Part model, mm, in its own coordinate system. Round coordinates to 2 decimals unless told otherwise and drop trailing zeros. Loops run counter-clockwise (first coordinate to the right, second up) from the corner with the lowest first, then second, coordinate; pieces in that order, holes last. Notation, with made-up numbers: (83, 28) - (98, 28) arc R19 cw to (98, 57) - close; hole circle Ø8 at (-5.75, 17.5). An arc over 180 degrees is marked (long way). Put each result on its own line as item: value.
from build123d import *

# Parameters (mm, degrees)
SKETCH_1_W          = 65
SKETCH_1_H          = 105
EXTRUDE_1_DEPTH     = 3
SKETCH_2_R          = 1.4
CUT_EXTRUDE_1_DEPTH = 62.818282085
SKETCH_3_R          = 1.4
CUT_EXTRUDE_2_DEPTH = 62.818282085
SKETCH_6_R          = 1.5
CUT_EXTRUDE_5_DEPTH = 62.818282085


with BuildPart() as part:
    # 草图1 → 凸台-拉伸1 (new body)
    with BuildSketch(Plane(origin=(0, 0, 0), x_dir=(1, 0, 0), z_dir=(0, 1, 0))):
        Rectangle(SKETCH_1_W, SKETCH_1_H)
    extrude(amount=EXTRUDE_1_DEPTH)

    # 草图2 → 切除-拉伸1 (cut, through all)
    with BuildSketch(Plane(origin=(0, 3, 0), x_dir=(1, 0, 0), z_dir=(0, 1, 0))):
        with Locations(Location((-28.1, -49.5, 0), (0, 0, 270))):
            Circle(SKETCH_2_R)
        with Locations(Location((28.1, -49.5, 0), (0, 0, 270))):
            Circle(SKETCH_2_R)
        with Locations(Location((28.1, -0.5, 0), (0, 0, 270))):
            Circle(SKETCH_2_R)
        with Locations(Location((-28.1, -0.5, 0), (0, 0, 270))):
            Circle(SKETCH_2_R)
    extrude(amount=-CUT_EXTRUDE_1_DEPTH, mode=Mode.SUBTRACT)

    # 草图3 → 切除-拉伸2 (cut, through all)
    with BuildSketch(Plane(origin=(0, 3, 0), x_dir=(1, 0, 0), z_dir=(0, 1, 0))):
        with Locations(Location((-16.7, 9.5, 0), (0, 0, 270))):
            Circle(SKETCH_3_R)
        with Locations(Location((28.1, 9.5, 0), (0, 0, 270))):
            Circle(SKETCH_3_R)
        with Locations(Location((28.1, 49.5, 0), (0, 0, 270))):
            Circle(SKETCH_3_R)
        with Locations(Location((-16.7, 49.5, 0), (0, 0, 270))):
            Circle(SKETCH_3_R)
    extrude(amount=-CUT_EXTRUDE_2_DEPTH, mode=Mode.SUBTRACT)

    # 草图6 → 切除-拉伸5 (cut, through all)
    with BuildSketch(Plane(origin=(0, 3, 0), x_dir=(1, 0, 0), z_dir=(0, 1, 0))):
        with Locations(Location((-20, -37.5, 0), (0, 0, 270))):
            Circle(SKETCH_6_R)
        with Locations(Location((20, -37.5, 0), (0, 0, 270))):
            Circle(SKETCH_6_R)
        with Locations(Location((20, 37.5, 0), (0, 0, 270))):
            Circle(SKETCH_6_R)
        with Locations(Location((-20, 37.5, 0), (0, 0, 270))):
            Circle(SKETCH_6_R)
    extrude(amount=-CUT_EXTRUDE_5_DEPTH, mode=Mode.SUBTRACT)


solid = part.part
1. Band-saw the part on A-A (x = 20). List the corners of the cut face in (y, z).
A:
outline: (0, -52.5) - (3, -52.5) - (3, -39) - (0, -39) - close; (0, -36) - (3, -36) - (3, 36) - (0, 36) - close; (0, 39) - (3, 39) - (3, 52.5) - (0, 52.5) - close
2. Probe line 1 along X through (y, z) = (0.9, -9.5); line 2 along X through (y, z) = (1.35, 0.5); line 3 along Z through (x, y) = (-28, 1.35). List the from-to ranges inside material, lowest first. Write a range as [from, to].
A:
line 1: x = [-32.5, -18.1], [-15.3, 26.7], [29.5, 32.5]
line 2: x = [-32.5, -29.5], [-26.7, 26.7], [29.5, 32.5]
line 3: z = [-52.5, -0.9], [1.9, 48.1], [50.9, 52.5]
3. Band-saw the part on B-B (z = 37.5). List the corners of the cut face in (x, y), plus the area to 3 significant figures.
A:
outline: (-32.5, 0) - (-21.5, 0) - (-21.5, 3) - (-32.5, 3) - close; (-18.5, 0) - (18.5, 0) - (18.5, 3) - (-18.5, 3) - close; (21.5, 0) - (32.5, 0) - (32.5, 3) - (21.5, 3) - close
area: 177 mm²
4. Two-plate mould, pull along Z, no slides. Class faces 1 (the cylindrical face through (-29.34, 1.52, 50.15)), 2 (the flat face through (0, 0, -1)), 3 (the flat face through (0, 1, -52.5)): pulls with the +Z half, pulls with the -Z half, needs draft (parallel to the pull), parting line crosses it, or undercut.
A:
face 1: undercut
face 2: needs draft
face 3: pulls with the -Z half
